Here's the drawing with two shaded views (mm, measured from the low corner). I have some questions. A direction names the side the tool comes from. Coordinates: 2 decimals unless noted, no trailing zeros. Write each loop counter-clockwise with the first axis right and the second up, starting at its lowest first coordinate (ties: lowest second). Pieces come first, ordered by that corner, then holes.
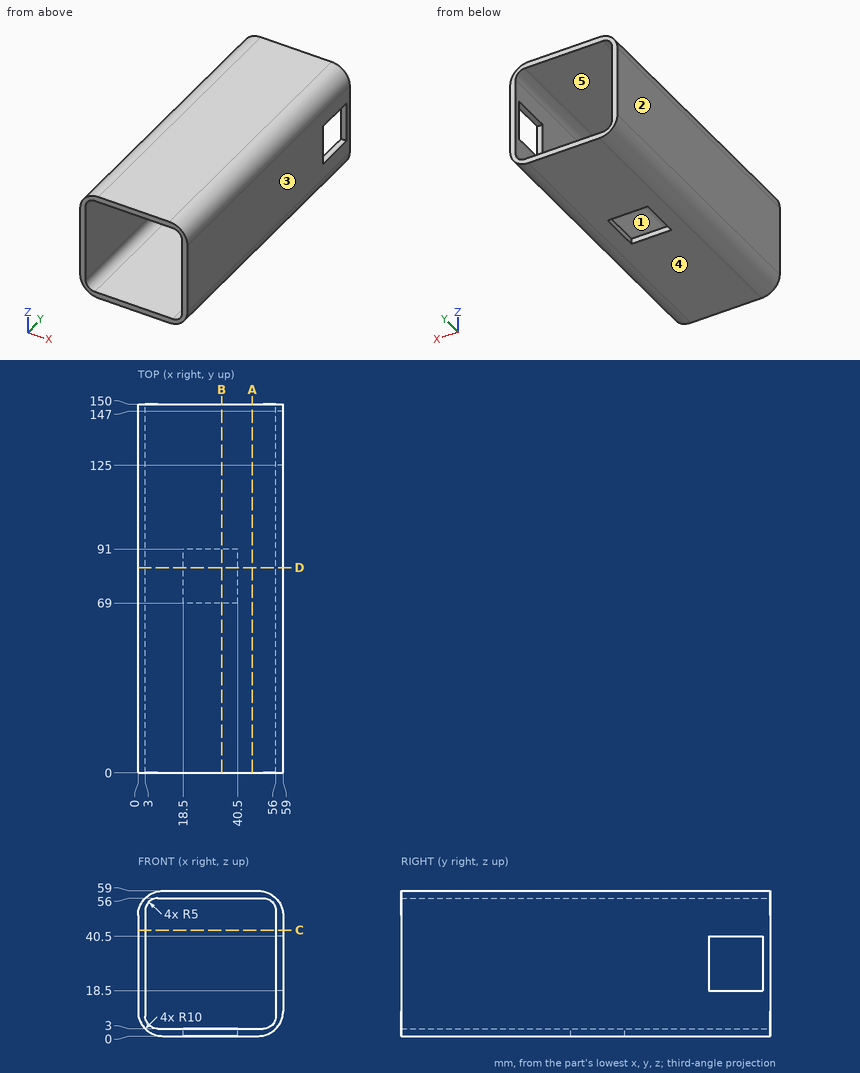
1. If we mould it in two halves opening along X, with no side actions, what happens to the marked faces 3, 4 and 5? For each: pulls with the +X half, pulls with the -X half, needs draft (parallel to the pull), parting line crosses it, or undercut.
Verdict:
face 3: pulls with the +X half
face 4: needs draft
face 5: undercut
2. I want a section at C-C on z = 43. Please give me the cut outline in (x, y).
Verdict:
outline: (0, 0) - (3, 0) - (3, 150) - (0, 150) - close; (56, 0) - (59, 0) - (59, 150) - (56, 150) - close
3. I want a section at A-A on x = 46.5. Please give me the cut outline in (y, z).
Verdict:
outline: (0, 0) - (150, 0) - (150, 3) - (0, 3) - close; (0, 56) - (150, 56) - (150, 59) - (0, 59) - close
4. I want a section at D-D on y = 83.5. Please give me the cut outline in (x, z).
Verdict:
outline: (0, 10) arc R10 ccw to (10, 0) - (18.5, 0) - (18.5, 3) - (8, 3) arc R5 cw to (3, 8) - (3, 51) arc R5 cw to (8, 56) - (51, 56) arc R5 cw to (56, 51) - (56, 8) arc R5 cw to (51, 3) - (40.5, 3) - (40.5, 0) - (49, 0) arc R10 ccw to (59, 10) - (59, 49) arc R10 ccw to (49, 59) - (10, 59) arc R10 ccw to (0, 49) - close
5. I want a section at B-B on x = 34. Please give me the cut outline in (y, z).
Verdict:
outline: (0, 0) - (69, 0) - (69, 3) - (0, 3) - close; (0, 56) - (150, 56) - (150, 59) - (0, 59) - close; (91, 0) - (150, 0) - (150, 3) - (91, 3) - close
6. For pin 1 (2.5 mm diameter, centred on y = 78, z = 1.5, fed in from +X); pin 2 (2.5 mm diameter, centred on x = 57, y = 137.5, fed in from -Z); pin 3 (3.5 mm diameter, centred on y = 85, z = 1.5, fed in from -X), each with a flat end and sliding along its axis, tell me the tip position at first contact or that it passes through.
Verdict:
pin 1: stops at x = 55.89
pin 2: stops at z = 2.62
pin 3: stops at x = 2.62
7. Please list where these lines run through material, in increasing order: line 1 along X through (y, z) = (13, 13); line 2 along X through (y, z) = (119.5, 54).
Verdict:
line 1: x = 0 to 3, 56 to 59
line 2: x = 1.34 to 4, 55 to 57.66
8. On a 3-axis mill with a long thin cutter (end or side, diameter ignored), from which of +Z, -Z, +X, -X, +Y, -Y can I reach the whole of each face in a straight line? I mean the marked faces 1 and 2. Say none if no direction works.
Verdict:
face 1: +Y, -Y
face 2: +Z, -Z, -X, +Y, -Y
